Input: part model. Units: mm. Frame: model coordinates. Give positions to 0.01 mm unless a question says otherwise; leave off trailing zeros. Order: outer loops, then holes, each group sorted by start corner. A loop starts at its lowest first (then second) coordinate and runs counter-clockwise, first axis right, second up. Notation, with made-up numbers: M 29.5,-40 L 36.5,-40 A25 ccw 36.5,-5 Z; hole C -29,-22.5 d6. An arc over 180 degrees is marked long. Use a Markdown table: item, result.
Autodesk Fusion 360 part; units mm, degrees
sketch "Sketch1" plane through (0, 0, 0) normal (0, 0, 1) x (1, 0, 0)
  line L0 (0, 0) -> (75, 0)
  line L1 (75, 0) -> (75, 30)
  line L2 (75, 30) -> (0, 30)
  line L3 (0, 30) -> (0, 0)
extrude "Extrude1" add sketch "Sketch1" along normal blind 5
hole "Hole1" at (16.3939, 15.4301, 5) direction (0, 0, -1) diameter 12.023 depth 10 tip angle 180
1) Cut plane C-C on z = 1.55. Return loops of the section in (x, y), and give its area (3 significant figures).
Response values:
| item | result |
|---|---|
| outline | M 0,0 L 75,0 L 75,30 L 0,30 Z; hole C 16.39,15.43 d12.02 |
| area | 2,140 mm² |
2) Cut plane A-A on x = 14. Return loops of the section in (y, z), and give its area (3 significant figures).
Response values:
| item | result |
|---|---|
| outline | M 0,0 L 9.92,0 L 9.92,5 L 0,5 Z; M 20.94,0 L 30,0 L 30,5 L 20.94,5 Z |
| area | 94.9 mm² |
3) Mould query, pull axis Y, two halves, no side actions, for faces 1 (the face through (38, 30, 2)), 2 (the face through (18.7, 9.88, 2.46)), 3 (the face through (37, 0, 2)), 4 (the face through (0, 15, 2)). Classes: released by +Y, released by -Y, zero draft, split by the parting line, or undercut.
Response values:
| item | result |
|---|---|
| face 1 | released by +Y |
| face 2 | undercut |
| face 3 | released by -Y |
| face 4 | zero draft |
4) Material intervals for line 1 (X direction, y = 14.25, z = 4.6); line 2 (Y direction, x = 16.5, z = 1.05); line 3 (X direction, y = 13.25, z = 1.9), sorted ascending. Write a range as from..to.
Response values:
| item | result |
|---|---|
| line 1 | x = 0..10.5, 22.29..75 |
| line 2 | y = 0..9.42, 21.44..30 |
| line 3 | x = 0..10.79, 22..75 |
5) Cut plane B-B on y = 11.5. Return loops of the section in (x, z) (3 decimals), and give its area (3 significant figures).
Response values:
| item | result |
|---|---|
| outline | M 0,0 L 11.845,0 L 11.845,5 L 0,5 Z; M 20.943,0 L 75,0 L 75,5 L 20.943,5 Z |
| area | 330 mm² |
